from build123d import *

# Parameters (mm, degrees)
F1_R     = 4.072632
F2_DEPTH = 7.62
F3_D     = 6.985
F4_R     = 4.013855
F5_DEPTH = 2.54


with BuildPart() as f2:
    # F1 (on Top) → F2 (new body)
    with BuildSketch(Plane.XY):
        Circle(F1_R)
    extrude(amount=F2_DEPTH)

    # F3 (through all)
    with Locations(Plane(origin=(0, 0, 0), x_dir=(1, 0, 0), z_dir=(0, 0, -1))):
        with Locations((0, 0)):
            Hole(F3_D / 2)

    # F4 (on Top) → F5 (join)
    with BuildSketch(Plane.XY):
        Circle(F4_R)
    extrude(amount=F5_DEPTH)


solid = f2.part
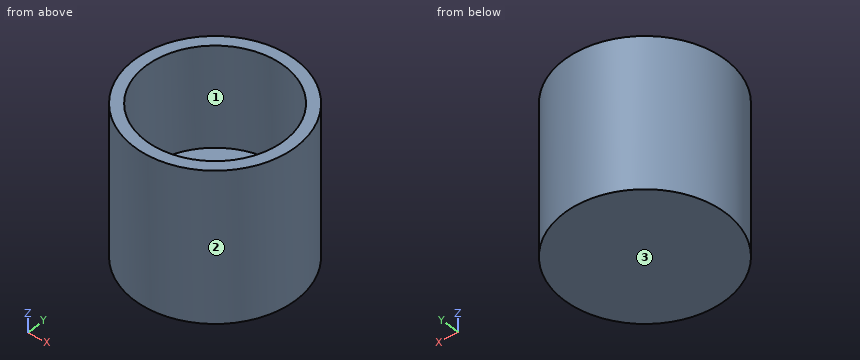
Here's how the part is built. I have some questions about the finished solid (model axes, mm). Face numbers are marked on the shaded views. Give positions to 0.01 mm unless a question says otherwise; leave off trailing zeros. Write each loop counter-clockwise with the first axis right and the second up, starting at its lowest first coordinate (ties: lowest second). Pieces come first, ordered by that corner, then holes. Notation, with made-up numbers: (36, -19) -> (55, -19) arc R18 ccw to (55, -1) -> close; hole circle Ø4 at (43.25, 81). An arc over 180 degrees is marked (long way). Use one line per item in the form item = value. Start each with the question number.
1. Imagine slicing it at D-D on z = 1.75. List the corners of the cut face in (x, y) for me.
2. If I drill on L1, parallel to Y at x = 0, z = 6.55; L2, parallel to Z at x = 3.25, y = -0.75; L3, parallel to X at y = 1.75, z = 3.75, over which ranges is the centre line in solid material (lowest first)?
3. Will these pins go through, and if not, where does the flat tip stop? pin 1 Ø1.5 at (x, y) = (-2, 2.5) entering from +Z; pin 2 Ø1.5 at (y, z) = (-1.5, 4) entering from -X; pin 3 Ø3.5 at (x, y) = (0, 1) entering from +Z.
4. Thinking about a two-plate mould opening in X: for the marked faces 1, 2 and 3, which applies, +X half, -X half, draft (parallel to the pull), parting line (faces both ways), or undercut?
5. Imagine slicing it at A-A on x = 0. List the corners of the cut face in (y, z) for me.
6. Imagine slicing it at B-B on z = 6.25. List the corners of the cut face in (x, y) for me (1 decimal), plus the area to 3 significant figures.
Entries:
q1.outline = circle Ø8.15 at (0, 0)
q2.L1 = -4.07 to -3.49, 3.49 to 4.07
q2.L2 = 0 to 2.54
q2.L3 = -3.68 to -3.02, 3.02 to 3.68
q3.pin_1 = 7.62
q3.pin_2 = -4
q3.pin_3 = 2.54
q4.face_1 = undercut
q4.face_2 = parting line
q4.face_3 = draft
q5.outline = (-4.07, 0) -> (4.07, 0) -> (4.07, 7.62) -> (3.49, 7.62) -> (3.49, 2.54) -> (-3.49, 2.54) -> (-3.49, 7.62) -> (-4.07, 7.62) -> close
q6.outline = circle Ø8.1 at (0, 0); hole circle Ø7 at (0, 0)
q6.area = 13.8 mm²
